Model file for the job. Use its own axes, mm. Coordinates: 2 decimals unless noted, no trailing zeros. Write each loop counter-clockwise with the first axis right and the second up, starting at its lowest first coordinate (ties: lowest second). Pieces come first, ordered by that corner, then holes. Notation, with made-up numbers: (-3.75, 84) -> (41.25, 84) arc R13 cw to (41.25, 102) -> close; hole circle Ø7 at (-1, -30). An arc over 180 degrees is marked (long way). Answer as a JSON object with one key per item and string values. Group by question number.
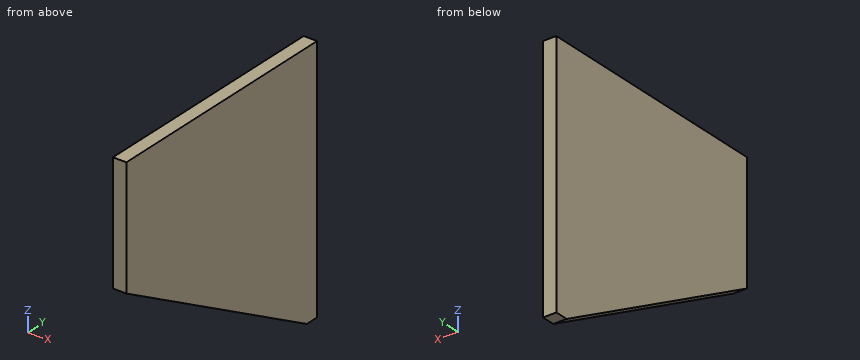
from build123d import *

# Parameters (mm, degrees)
SALIENTE_EXTRUIR1_DEPTH = 20


with BuildPart() as part:
    # Croquis2 → Saliente-Extruir1 (new body)
    with BuildSketch(Plane.ZY.offset(192.754092983)):
        Polygon((360, 202.834413862), (360, -167.165586138), (182, -167.165586138), (-15, 182.834413862), (-15, 202.834413862), align=None)
    extrude(amount=-SALIENTE_EXTRUIR1_DEPTH)


solid = part.part
(1) Pin check, flat tips, straight feed: pin 1 (12 mm diameter, centred on x = -185, z = 44.5, fed in from -Y); pin 2 (1 mm diameter, centred on x = -183, y = 18.5, fed in from -Z); pin 3 (3 mm diameter, centred on x = -189, y = -103, fed in from -Z). Stop position of each tip, or through.
(2) Wall check: probe 1 along Y at (x, z) = (-188, 172.5); probe 2 along Z at (x, y) = (-182.5, 177); probe 3 along Z at (x, y) = (-188.5, 15.5). Give the ranges that are in metal, low to high.
(3) Cut at B-B on z = 113.5. List the corners of the cut face in (x, y).
(4) Cut at C-C on y = -140.5. List the corners of the cut face in (x, z), plus the area to 3 significant figures.
(5) Cut at A-A on x = -181.5. List the corners of the cut face in (y, z), plus the area to 3 significant figures.
Results found:
{
 "1": {"pin 1": "stops at y = 66.46", "pin 2": "stops at z = 77.22", "pin 3": "stops at z = 145.04"},
 "2": {"probe 1": "y = -150.29 to 202.83", "probe 2": "z = -11.72 to 360", "probe 3": "z = 79.19 to 360"},
 "3": {"outline": "(-192.75, -45.47) -> (-172.75, -45.47) -> (-172.75, 202.83) -> (-192.75, 202.83) -> close"},
 "4": {"outline": "(-192.75, 166.99) -> (-172.75, 166.99) -> (-172.75, 360) -> (-192.75, 360) -> close", "area": "3,860 mm²"},
 "5": {"outline": "(-167.17, 182) -> (182.83, -15) -> (202.83, -15) -> (202.83, 360) -> (-167.17, 360) -> close", "area": "104,000 mm²"}
}
